Read the model definition and answer for the solid it produces. Units are mm, in the model's axes. A direction names the side the tool comes from. Coordinates: 2 decimals unless noted, no trailing zeros. Write each loop counter-clockwise with the first axis right and the second up, starting at its lowest first coordinate (ties: lowest second). Pieces come first, ordered by that corner, then holes. Notation, with made-up numbers: (56.5, -31.75) - (97.5, -31.75) arc R22 ccw to (97.5, -9.75) - close; hole circle Ø11 at (73, 79.5). An arc over 180 degrees is marked (long way). Return JSON: item names as keys, results as strings.
Autodesk Inventor part; units mm, degrees
ref_plane "YZ Plane" through (0, 0, 0) normal (1, 0, 0) x (0, 1, 0)
ref_plane "XZ Plane" through (0, 0, 0) normal (0, 1, 0) x (-1, 0, 0)
ref_plane "XY Plane" through (0, 0, 0) normal (0, 0, 1) x (1, 0, 0)
sketch "Sketch1" plane through (0, 0, 0) normal (0, 1, 0) x (-1, 0, 0)
  line L0 (0, 0) -> (0, 182) construction
  line L1 (0, 182) -> (51.8, 182) construction
  line L2 (51.8, 182) -> (51.8, 91)
  line L3 (51.8, 91) -> (55, 91)
  line L4 (55, 91) -> (55, 0)
  line L5 (55, 0) -> (58.2, 0)
  line L6 (58.2, 0) -> (58.2, 182)
  line L7 (58.2, 182) -> (51.8, 182)
  line L8 (55, 0) -> (0, 0) construction
  line L9 (0, 182) -> (0, 385) construction
  line L10 (0, 385) -> (-143.5427, 528.5427) construction
  line L11 (-143.5427, 528.5427) -> (-106.9145, 565.1708) construction
  line L12 (-106.9145, 565.1708) -> (-171.2215, 629.4777)
  line L13 (-171.2215, 629.4777) -> (-168.9587, 631.7405)
  line L14 (-168.9587, 631.7405) -> (-233.3452, 696.127)
  line L15 (-233.3452, 696.127) -> (-231.0825, 698.3897)
  line L16 (-231.0825, 698.3897) -> (-102.3891, 569.6963)
  line L17 (-106.9145, 565.1708) -> (-102.3891, 569.6963)
  line L18 (-143.5427, 528.5427) -> (-272.2361, 657.2361) construction
  line L19 (-233.3452, 696.127) -> (-272.2361, 657.2361) construction
  line L20 (0, 182) -> (-490.0854, 182) construction
  line L21 (-143.5427, 528.5427) -> (-490.0854, 182) construction
  arc A0 (0, 182) -> (-143.5427, 528.5427) centre (-490.0854, 182) ccw
  line L22 (-143.5427, 528.5427) -> (-143.5427, 182) construction
  line L23 (51.8, 91) -> (0, 91) construction
  line L24 (-171.2215, 629.4777) -> (-207.8496, 592.8496) construction
  dimension "d0" = 182
  dimension "d1" = 91
  dimension "d2" = 103.6
  dimension "d3" = 110
  dimension "d4" = 116.4
  dimension "d5" = 203
  dimension "d6" = 203
  dimension "d7" = 182
  dimension "d8" = 91
  dimension "d9" = 103.6
  dimension "d10" = 110
  dimension "d11" = 116.4
  dimension "d12" = 45
revolve "Revolve1" add sketch "Sketch1" angle 360 about axis through (0, 0, 0) along (0, 0, 1) contours L7 L6 L5 L4 L3 L2
revolve "Revolve2" add sketch "Sketch1" angle 360 about axis through (143.5427, 0, 528.5427) along (0.7071068, 0, 0.7071068) contours L12 L13 L14 L15 L16 L17
sketch "Sketch2" plane through (0, 0, 182) normal (0, 0, 1) x (1, 0, 0)
  circle A0 centre (0, 0) radius 51.8
  circle A1 centre (0, 0) radius 55
sweep "Sweep1" add profiles "Sketch2" path "Sketch1" path curves A0
equation "\"d0\" = 2 * tk"
equation "\"d1\" = tk"
equation "\"d2\" = d - 2 * s1"
equation "\"d3\" = d"
equation "\"d4\" = d + 2 * s1"
equation "\"d5\" = zk"
equation "\"d6\" = zk"
equation "\"d7\" = 2 * tk"
equation "\"d8\" = tk"
equation "\"d9\" = d - 2 * s1"
equation "\"d10\" = d"
equation "\"d11\" = d + 2 * s1"
equation "\"zk\" = 203"
equation "\"tk\" = 91"
equation "\"d\" = 110"
equation "\"s1\" = 3.2"
properties part number "DIN 8063 Двойная подвижная соединительная муфта с изгибом 45 градусов со стыковой сваркой - MMK - KK 110 - 3" material "ПВХ, непластифицированный"
(1) Which of the six approach directions +Z, -Z, +X, -X, +Y, -Y give full straight-line access (tool end or side, diameter ignored) to faces 1 (the face through (11.23, -50.57, 135.86)), 2 (the face through (222.1, 48.6, 578.6))?
Answer:
{"face 1": "-Z", "face 2": "none"}
(2) Flat-ended cylindrical pins translate along their axes: P1, Ø1.5, axis at y = 8, z = 547.5, coming from the +X side; P2, Ø1.5, axis at x = 189, y = -17.5, coming from the +Z side; P3, Ø6, axis at x = 120, y = -1, coming from the +Z side. Find the tip coordinate at first contact, or state that the pin passes through.
Answer:
{"P1": "x = 244.79", "P2": "z = 653.32", "P3": "z = 590.3"}
(3) A cutting plane is placed at A-A (z = 83). Determine the outline of the cut face in (x, y), and give its area (3 significant figures).
Answer:
{"outline": "circle Ø116.4 at (0, 0); hole circle Ø110 at (0, 0)", "area": "1,140 mm²"}
(4) Determine the mould class of faces 3 (the face through (302.53, -34.76, 626.94)), 4 (the face through (182.537, -2.427, 489.548)), 5 (the face through (35, 43, 0)) for opening direction X: +X half, -X half, draft (parallel to the pull), parting line (faces both ways), or undercut.
Answer:
{"face 3": "+X half", "face 4": "undercut", "face 5": "draft"}
(5) Straight lines are drawn through the part: line 1 (Y direction, x = 0, z = 37); line 2 (Y direction, x = 0, z = 125). For each, find the intervals that lie inside material, in ascending order. Write a range as from..to.
Answer:
{"line 1": "-58.2..-55, 55..58.2", "line 2": "-58.2..-51.8, 51.8..58.2"}
